Autodesk Inventor part; units mm, degrees
ref_plane "YZ Plane" through (0, 0, 0) normal (1, 0, 0) x (0, 1, 0)
ref_plane "XZ Plane" through (0, 0, 0) normal (0, 1, 0) x (-1, 0, 0)
ref_plane "XY Plane" through (0, 0, 0) normal (0, 0, 1) x (1, 0, 0)
sketch "Sketch1" plane through (0, 0, 0) normal (0, 0, 1) x (1, 0, 0)
  line L0 (-10, -10) -> (-5.6, -10)
  line L1 (-10, -5.6) -> (-10, -10)
  line L2 (-5.6, -10) -> (-5, -10)
  line L3 (-3.2, -8.2) -> (-5.6, -8.2)
  line L4 (-2.8351, -3.825) -> (-5.6, -6.5899)
  line L5 (-3.825, -2.8351) -> (-6.5899, -5.6)
  line L6 (0, 0) -> (0, -11) construction
  line L7 (0, 0) -> (-12, 0) construction
  line L8 (-3.2, -8.2) -> (-5, -10)
  line L9 (-6.5899, -5.6) -> (-8.2, -5.6)
  line L10 (-10, -5.6) -> (-10, -5)
  line L11 (-10, -5) -> (-8.2, -3.2)
  line L12 (-8.2, -3.2) -> (-8.2, -5.6)
  line L13 (-5.6, -8.2) -> (-5.6, -6.5899)
  arc A0 (-2.15, 0) -> (0, -2.15) centre (0, 0) ccw
  line L14 (0, 0) -> (-3.825, 0)
  line L15 (-3.825, 0) -> (-3.825, -2.8351)
  line L16 (-2.8351, -3.825) -> (0, -3.825)
  line L17 (0, -3.825) -> (0, 0)
  line L18 (-2.8351, -3.825) -> (-3.825, -3.825) construction
  line L19 (-3.825, -3.825) -> (-3.825, -2.8351) construction
  line L20 (3.825, -2.8351) -> (3.825, -3.825) construction
  line L21 (3.825, -2.8351) -> (3.825, 0)
  line L22 (3.825, -3.825) -> (2.8351, -3.825) construction
  line L23 (3.825, 0) -> (0, 0)
  line L24 (0, -3.825) -> (2.8351, -3.825)
  arc A1 (0, -2.15) -> (2.15, 0) centre (0, 0) ccw
  line L25 (0, 0) -> (0, -3.825)
  line L26 (2.8351, -3.825) -> (5.6, -6.5899)
  line L27 (0, 0) -> (0, -12) construction
  line L28 (0, 0) -> (11, 0) construction
  line L29 (3.825, -2.8351) -> (6.5899, -5.6)
  line L30 (8.2, -3.2) -> (8.2, -5.6)
  line L31 (10, -5.6) -> (10, -5)
  line L32 (8.2, -3.2) -> (10, -5)
  line L33 (8.2, -5.6) -> (6.5899, -5.6)
  line L34 (5.6, -6.5899) -> (5.6, -8.2)
  line L35 (10, -10) -> (10, -5.6)
  line L36 (5.6, -10) -> (10, -10)
  line L37 (3.2, -8.2) -> (5.6, -8.2)
  line L38 (5, -10) -> (3.2, -8.2)
  line L39 (5.6, -10) -> (5, -10)
  line L40 (2.8351, 3.825) -> (3.825, 3.825) construction
  line L41 (2.8351, 3.825) -> (0, 3.825)
  line L42 (3.825, 3.825) -> (3.825, 2.8351) construction
  line L43 (0, 3.825) -> (0, 0)
  line L44 (3.825, 0) -> (3.825, 2.8351)
  arc A2 (2.15, 0) -> (0, 2.15) centre (0, 0) ccw
  line L45 (0, 0) -> (3.825, 0)
  line L46 (3.825, 2.8351) -> (6.5899, 5.6)
  line L47 (0, 0) -> (12, 0) construction
  line L48 (0, 0) -> (0, 11) construction
  line L49 (2.8351, 3.825) -> (5.6, 6.5899)
  line L50 (3.2, 8.2) -> (5.6, 8.2)
  line L51 (5.6, 10) -> (5, 10)
  line L52 (3.2, 8.2) -> (5, 10)
  line L53 (5.6, 8.2) -> (5.6, 6.5899)
  line L54 (6.5899, 5.6) -> (8.2, 5.6)
  line L55 (10, 10) -> (5.6, 10)
  line L56 (10, 5.6) -> (10, 10)
  line L57 (8.2, 3.2) -> (8.2, 5.6)
  line L58 (10, 5) -> (8.2, 3.2)
  line L59 (10, 5.6) -> (10, 5)
  line L60 (-3.825, 2.8351) -> (-3.825, 3.825) construction
  line L61 (-3.825, 2.8351) -> (-3.825, 0)
  line L62 (-3.825, 3.825) -> (-2.8351, 3.825) construction
  line L63 (-3.825, 0) -> (0, 0)
  line L64 (0, 3.825) -> (-2.8351, 3.825)
  arc A3 (0, 2.15) -> (-2.15, 0) centre (0, 0) ccw
  line L65 (0, 0) -> (0, 3.825)
  line L66 (-2.8351, 3.825) -> (-5.6, 6.5899)
  line L67 (0, 0) -> (0, 12) construction
  line L68 (0, 0) -> (-11, 0) construction
  line L69 (-3.825, 2.8351) -> (-6.5899, 5.6)
  line L70 (-8.2, 3.2) -> (-8.2, 5.6)
  line L71 (-10, 5.6) -> (-10, 5)
  line L72 (-8.2, 3.2) -> (-10, 5)
  line L73 (-8.2, 5.6) -> (-6.5899, 5.6)
  line L74 (-5.6, 6.5899) -> (-5.6, 8.2)
  line L75 (-10, 10) -> (-10, 5.6)
  line L76 (-5.6, 10) -> (-10, 10)
  line L77 (-3.2, 8.2) -> (-5.6, 8.2)
  line L78 (-5, 10) -> (-3.2, 8.2)
  line L79 (-5.6, 10) -> (-5, 10)
  point P0 (0, 2.15)
  point P1 (2.15, 0)
  point P2 (0, -2.15)
  dimension "d16" = 10
  dimension "d19" = 3.2
  dimension "d21" = 4.4
  dimension "d22" = 4.4
  dimension "d24" = 45
  dimension "d25" = 1.8
  dimension "d27" = 1.8
  dimension "d28" = 45
  dimension "d29" = 3.2
  dimension "d31" = 1.4
  dimension "d33" = 2.15
  dimension "d34" = 3.825
  dimension "d35" = 3.825
  dimension "d36" = 135
  dimension "d39" = 360
extrude "Extrusion1" add sketch "Sketch1" along normal blind 230 contours L1 L10 L11 L12 L9 L5 L15 L14 A0 L17 L16 L4 L13 L3 L8 L2 L0 | L17 A1 L23 L21 L29 L33 L30 L32 L31 L35 L36 L39 L38 L37 L34 L26 L24 | L61 L69 L73 L70 L72 L71 L75 L76 L79 L78 L77 L74 L66 L64 L43 A3 L14 | A2 L43 L41 L49 L53 L50 L52 L51 L55 L56 L59 L58 L57 L54 L46 L44 L23
properties part number "AP20x20"
CAD build for the part. Positions are in the model's coordinates, mm. A direction names the side the tool comes from. Give positions to 0.01 mm unless a question says otherwise; leave off trailing zeros. Order: outer loops, then holes, each group sorted by start corner. A loop starts at its lowest first (then second) coordinate and runs counter-clockwise, first axis right, second up.
(1) Saw through at A-A, the plane x = 0. Give the cut face in (y, z) (3 decimals), then the cut area to 4 significant figures.
(2) Drill centre lines: L1, parallel to X at y = -6, z = 125; L2, parallel to Y at x = 0, z = 50.5 (3 decimals). Where is each one in solid material? Low to high.
(3) Tool access for faces 1 (the flat face through (0, -3.825, 113)), 2 (the flat face through (10, 7, 113)), 3 (the flat face through (-3.825, 0, 113)): list every direction of +Z, -Z, +X, -X, +Y, -Y with a clear straight run to the whole face (end or side of a thin tool).
(4) Flat gauge pins, fed straight in: pin 1 (0.7 mm diameter, centred on y = 4.5, z = 89, fed in from -X); pin 2 (1 mm diameter, centred on x = 1, y = -7.5, fed in from +Z); pin 3 (1.7 mm diameter, centred on x = 0.5, z = 171, fed in from +Y) (3 decimals); pin 4 (6 mm diameter, centred on x = -1, z = 148, fed in from -Y). Where does each tip first touch, or does it go through?
(5) Mould opens along X. For faces 4 (the flat face through (3.825, 0, 113)), 5 (the flat face through (0, 3.825, 113)), 6 (the flat face through (-0.1, 2.4, 0)) say: released by +X, released by -X, zero draft, split by the parting line, or undercut.
Results found:
1. outline: (-3.825, 0) - (-2.15, 0) - (-2.15, 230) - (-3.825, 230) - close; (2.15, 0) - (3.825, 0) - (3.825, 230) - (2.15, 230) - close
1. area: 770.5 mm2
2. L1: x = -10 to -5.01, 5.01 to 10
2. L2: y = -3.825 to -2.15, 2.15 to 3.825
3. face 1: +Z, -Z, -Y
3. face 2: +Z, -Z, +X, +Y, -Y
3. face 3: +Z, -Z, -X
4. pin 1: stops at x = -9.85
4. pin 2: passes through
4. pin 3: stops at y = 3.825
4. pin 4: stops at y = -9
5. face 4: released by +X
5. face 5: undercut
5. face 6: zero draft
